Work out the finished part from the listing and answer in its coordinate system (mm). A direction names the side the tool comes from. Give positions to 0.01 mm unless a question says otherwise; leave off trailing zeros. Write each loop counter-clockwise with the first axis right and the second up, starting at its lowest first coordinate (ties: lowest second). Pieces come first, ordered by that corner, then holes.
1) Determine the mould class of faces 5 (the face through (-19.05, 0, 65)), 6 (the face through (23.59, 23.49, 67.05)), 7 (the face through (25.4, 0, 66)) for opening direction Y: pulls with the +Y half, pulls with the -Y half, needs draft (parallel to the pull), parting line crosses it, or undercut.
2) Find section A-A (z = 103.5). Determine the outline of the cut face in (x, y).
3) A tool of negligible diameter and unlimited length cuts with its end or side. For faces 1 (the face through (35, -2, 133)), 2 (the face through (-35, -2, 133)), 3 (the face through (-17.24, 17.14, 66.06)), 4 (the face through (-23.49, 23.59, 67.05)), from which of +Z, -Z, +X, -X, +Y, -Y can it reach the whole face along a straight path? Write none if from no direction.
4) Find section D-D (y = 1.5). Determine the outline of the cut face in (x, z).
5) Given pin 1 Ø11.5 at (x, z) = (-2.5, 87) entering from +Y; pin 2 Ø9.5 at (x, z) = (24, -8.5) entering from +Y; pin 3 Ø13 at (x, z) = (0, -8) entering from -Y; pin 4 Ø11 at (x, y) = (-53, 22.5) entering from +Z, each flat-ended and moving along its own axis, determine where each tip first touches the part or whether it passes through.
6) Find section B-B (x = 53). Determine the outline of the cut face in (y, z), plus the area to 3 significant figures.
7) Find section C-C (y = 22.5). Determine the outline of the cut face in (x, z), plus the area to 3 significant figures.
8) Straight lines are drawn through the part: probe 1 along Y at (x, z) = (-53, -8); probe 2 along X at (y, z) = (2, 120.5); probe 3 along X at (y, z) = (-22, -3). For each, find the intervals that lie inside material, in ascending order.
```python
from build123d import *

# Parameters (mm, degrees)
F0_W     = 130
F0_H     = 75
F1_DEPTH = 12
F3_DEPTH = 136
F5_D     = 12
F7_DEPTH = 50.8
F8_W     = 70
F8_H     = 90
F9_DEPTH = 12


with BuildPart() as f1:
    # F0 (on Top) → F1 (new body)
    with BuildSketch(Plane.XY):
        Rectangle(F0_W, F0_H)
    extrude(amount=-F1_DEPTH)

    # F2 (on face) → F3 (join)
    with BuildSketch(Plane.XY):
        with BuildLine():
            Line((-19.05, -25.4), (19.05, -25.4))
            ThreePointArc((19.05, -25.4), (23.5401280605, -23.5401280605), (25.4, -19.05))
            Line((25.4, -19.05), (25.4, 19.05))
            ThreePointArc((25.4, 19.05), (23.5401280605, 23.5401280605), (19.05, 25.4))
            Line((19.05, 25.4), (-19.05, 25.4))
            ThreePointArc((-19.05, 25.4), (-23.5401280605, 23.5401280605), (-25.4, 19.05))
            Line((-25.4, 19.05), (-25.4, -19.05))
            ThreePointArc((-25.4, -19.05), (-23.5401280605, -23.5401280605), (-19.05, -25.4))
        make_face()
        with BuildLine():
            Line((-12.7, 19.05), (12.7, 19.05))
            ThreePointArc((12.7, 19.05), (17.1901280605, 17.1901280605), (19.05, 12.7))
            Line((19.05, 12.7), (19.05, -12.7))
            ThreePointArc((19.05, -12.7), (17.1901280605, -17.1901280605), (12.7, -19.05))
            Line((12.7, -19.05), (-12.7, -19.05))
            ThreePointArc((-12.7, -19.05), (-17.1901280605, -17.1901280605), (-19.05, -12.7))
            Line((-19.05, -12.7), (-19.05, 12.7))
            ThreePointArc((-19.05, 12.7), (-17.1901280605, 17.1901280605), (-12.7, 19.05))
        make_face(mode=Mode.SUBTRACT)
    extrude(amount=F3_DEPTH)

    # F5 (through all)
    with Locations(Plane.XY):
        with Locations((-53, 22.5), (53, 22.5), (53, -22.5), (-53, -22.5)):
            Hole(F5_D / 2)

    # F6 (on face) → F7 (cut)
    with BuildSketch(Plane.YZ.offset(25.4)):
        Polygon((-19.05, 136), (-25.4, 136), (-25.4, 119.9340696072), (-19.05, 121.9423109063), align=None)
        Polygon((19.05, 136), (-19.05, 136), (-19.05, 121.9423109063), (19.05, 133.9917587009), align=None)
        Polygon((25.4, 136), (19.05, 136), (19.05, 133.9917587009), align=None)
    extrude(amount=-F7_DEPTH, mode=Mode.SUBTRACT)

    # F8 (on face) → F9 (join)
    with BuildSketch(Plane(origin=(0, -36.7908585502, 116.331614084), x_dir=(1, 0, 0), z_dir=(0, -0.3015379599, 0.9534541723))):
        with Locations((0, 38.5869186148)):
            Rectangle(F8_W, F8_H)
        with BuildLine():
            Line((25.4, 58.5669035507), (25.4, 18.6069336789))
            add(Edge.make_bspline(
                [(25.4, 18.6069336789), (25.4, 11.9469387003), (19.05, 11.9469387003)],
                knots=[4.7123889804, 4.7123889804, 4.7123889804, 6.2831853072, 6.2831853072, 6.2831853072], degree=2, weights=[1, 0.7071067812, 1]))
            Line((19.05, 11.9469387003), (-19.05, 11.9469387003))
            add(Edge.make_bspline(
                [(-19.05, 11.9469387003), (-25.4, 11.9469387003), (-25.4, 18.6069336789)],
                knots=[0, 0, 0, 1.5707963268, 1.5707963268, 1.5707963268], degree=2, weights=[1, 0.7071067812, 1]))
            Line((-25.4, 18.6069336789), (-25.4, 58.5669035507))
            add(Edge.make_bspline(
                [(-25.4, 58.5669035507), (-25.4, 65.2268985294), (-19.05, 65.2268985294)],
                knots=[1.5707963268, 1.5707963268, 1.5707963268, 3.1415926536, 3.1415926536, 3.1415926536], degree=2, weights=[1, 0.7071067812, 1]))
            Line((-19.05, 65.2268985294), (19.05, 65.2268985294))
            add(Edge.make_bspline(
                [(19.05, 65.2268985294), (25.4, 65.2268985294), (25.4, 58.5669035507)],
                knots=[3.1415926536, 3.1415926536, 3.1415926536, 4.7123889804, 4.7123889804, 4.7123889804], degree=2, weights=[1, 0.7071067812, 1]))
        make_face(mode=Mode.SUBTRACT)
        with BuildLine():
            add(Edge.make_bspline(
                [(25.4, 18.6069336789), (25.4, 11.9469387003), (19.05, 11.9469387003)],
                knots=[4.7123889804, 4.7123889804, 4.7123889804, 6.2831853072, 6.2831853072, 6.2831853072], degree=2, weights=[1, 0.7071067812, 1]))
            Line((25.4, 18.6069336789), (25.4, 58.5669035507))
            add(Edge.make_bspline(
                [(19.05, 65.2268985294), (25.4, 65.2268985294), (25.4, 58.5669035507)],
                knots=[3.1415926536, 3.1415926536, 3.1415926536, 4.7123889804, 4.7123889804, 4.7123889804], degree=2, weights=[1, 0.7071067812, 1]))
            Line((19.05, 65.2268985294), (-19.05, 65.2268985294))
            add(Edge.make_bspline(
                [(-25.4, 58.5669035507), (-25.4, 65.2268985294), (-19.05, 65.2268985294)],
                knots=[1.5707963268, 1.5707963268, 1.5707963268, 3.1415926536, 3.1415926536, 3.1415926536], degree=2, weights=[1, 0.7071067812, 1]))
            Line((-25.4, 58.5669035507), (-25.4, 18.6069336789))
            add(Edge.make_bspline(
                [(-19.05, 11.9469387003), (-25.4, 11.9469387003), (-25.4, 18.6069336789)],
                knots=[0, 0, 0, 1.5707963268, 1.5707963268, 1.5707963268], degree=2, weights=[1, 0.7071067812, 1]))
            Line((-19.05, 11.9469387003), (19.05, 11.9469387003))
        make_face()
        with BuildLine():
            Line((-19.05, 25.2669286576), (-19.05, 51.9069085721))
            add(Edge.make_bspline(
                [(-19.05, 51.9069085721), (-19.05, 58.5669035507), (-12.7, 58.5669035507)],
                knots=[1.5707963268, 1.5707963268, 1.5707963268, 3.1415926536, 3.1415926536, 3.1415926536], degree=2, weights=[1, 0.7071067812, 1]))
            Line((-12.7, 58.5669035507), (12.7, 58.5669035507))
            add(Edge.make_bspline(
                [(12.7, 58.5669035507), (19.05, 58.5669035507), (19.05, 51.9069085721)],
                knots=[3.1415926536, 3.1415926536, 3.1415926536, 4.7123889804, 4.7123889804, 4.7123889804], degree=2, weights=[1, 0.7071067812, 1]))
            Line((19.05, 51.9069085721), (19.05, 25.2669286576))
            add(Edge.make_bspline(
                [(19.05, 25.2669286576), (19.05, 18.6069336789), (12.7, 18.6069336789)],
                knots=[4.7123889804, 4.7123889804, 4.7123889804, 6.2831853072, 6.2831853072, 6.2831853072], degree=2, weights=[1, 0.7071067812, 1]))
            Line((12.7, 18.6069336789), (-12.7, 18.6069336789))
            add(Edge.make_bspline(
                [(-12.7, 18.6069336789), (-19.05, 18.6069336789), (-19.05, 25.2669286576)],
                knots=[0, 0, 0, 1.5707963268, 1.5707963268, 1.5707963268], degree=2, weights=[1, 0.7071067812, 1]))
        make_face(mode=Mode.SUBTRACT)
        with BuildLine():
            add(Edge.make_bspline(
                [(-19.05, 51.9069085721), (-19.05, 58.5669035507), (-12.7, 58.5669035507)],
                knots=[1.5707963268, 1.5707963268, 1.5707963268, 3.1415926536, 3.1415926536, 3.1415926536], degree=2, weights=[1, 0.7071067812, 1]))
            Line((-19.05, 51.9069085721), (-19.05, 25.2669286576))
            add(Edge.make_bspline(
                [(-12.7, 18.6069336789), (-19.05, 18.6069336789), (-19.05, 25.2669286576)],
                knots=[0, 0, 0, 1.5707963268, 1.5707963268, 1.5707963268], degree=2, weights=[1, 0.7071067812, 1]))
            Line((-12.7, 18.6069336789), (12.7, 18.6069336789))
            add(Edge.make_bspline(
                [(19.05, 25.2669286576), (19.05, 18.6069336789), (12.7, 18.6069336789)],
                knots=[4.7123889804, 4.7123889804, 4.7123889804, 6.2831853072, 6.2831853072, 6.2831853072], degree=2, weights=[1, 0.7071067812, 1]))
            Line((19.05, 25.2669286576), (19.05, 51.9069085721))
            add(Edge.make_bspline(
                [(12.7, 58.5669035507), (19.05, 58.5669035507), (19.05, 51.9069085721)],
                knots=[3.1415926536, 3.1415926536, 3.1415926536, 4.7123889804, 4.7123889804, 4.7123889804], degree=2, weights=[1, 0.7071067812, 1]))
            Line((12.7, 58.5669035507), (-12.7, 58.5669035507))
        make_face()
    extrude(amount=F9_DEPTH)


solid = f1.part
```
Results:
1. face 5: undercut
1. face 6: pulls with the +Y half
1. face 7: needs draft
2. outline: (-25.4, -19.05) arc R6.35 ccw to (-19.05, -25.4) - (19.05, -25.4) arc R6.35 ccw to (25.4, -19.05) - (25.4, 19.05) arc R6.35 ccw to (19.05, 25.4) - (-19.05, 25.4) arc R6.35 ccw to (-25.4, 19.05) - close; hole (-19.05, -12.7) arc R6.35 ccw to (-12.7, -19.05) - (12.7, -19.05) arc R6.35 ccw to (19.05, -12.7) - (19.05, 12.7) arc R6.35 ccw to (12.7, 19.05) - (-12.7, 19.05) arc R6.35 ccw to (-19.05, 12.7) - close
3. face 1: +Z, +X, +Y, -Y
3. face 2: +Z, -X, +Y, -Y
3. face 3: none
3. face 4: -X, +Y
4. outline: (-65, -12) - (65, -12) - (65, 0) - (25.4, 0) - (25.4, 128.44) - (35, 128.44) - (35, 141.03) - (-35, 141.03) - (-35, 128.44) - (-25.4, 128.44) - (-25.4, 0) - (-65, 0) - close; hole (-19.05, 0) - (19.05, 0) - (19.05, 128.44) - (-19.05, 128.44) - close
5. pin 1: stops at y = 25.4
5. pin 2: stops at y = 37.5
5. pin 3: stops at y = -37.5
5. pin 4: passes through
6. outline: (-37.5, -12) - (-28.5, -12) - (-28.5, 0) - (-37.5, 0) - close; (-16.5, -12) - (16.5, -12) - (16.5, 0) - (-16.5, 0) - close; (28.5, -12) - (37.5, -12) - (37.5, 0) - (28.5, 0) - close
6. area: 612 mm2
7. outline: (-65, -12) - (-59, -12) - (-59, 0) - (-65, 0) - close; (-47, -12) - (47, -12) - (47, 0) - (24.38, 0) - (24.38, 135.08) - (35, 135.08) - (35, 147.67) - (-35, 147.67) - (-35, 135.08) - (-24.38, 135.08) - (-24.38, 0) - (-47, 0) - close; (59, -12) - (65, -12) - (65, 0) - (59, 0) - close
7. area: 8,740 mm2
8. probe 1: y = -37.5 to -28.5, -16.5 to 16.5, 28.5 to 37.5
8. probe 2: x = -25.4 to -19.05, 19.05 to 25.4
8. probe 3: x = -65 to -58.98, -47.02 to 47.02, 58.98 to 65
